Model file for the job. Use its own axes, mm. Coordinates: 2 decimals unless noted, no trailing zeros. Write each loop counter-clockwise with the first axis right and the second up, starting at its lowest first coordinate (ties: lowest second). Pieces come first, ordered by that corner, then holes. Notation, with made-up numbers: M 88.5,33.25 L 133.5,33.25 A24 cw 133.5,65.25 Z; hole C 30.5,26.5 d2. An arc over 180 degrees is marked long. Put each result on its own line as item: value. Start each with the question number.
Q1. Pull direction Z, two halves, no side cores. Call faces 1 (the flat face through (58, 5, 0)), 2 (the cylindrical face through (37.253, -0.902, -0.121)), 3 (the flat face through (-1, 5, 18)): pulls with the +Z half, pulls with the -Z half, needs draft (parallel to the pull), parting line crosses it, or undercut.
Q2. Drop flat-ended pins along their axis: pin 1 (3.5 mm diameter, centred on x = -40, z = 0, fed in from +Y); pin 2 (2 mm diameter, centred on x = 40, y = 6, fed in from -Z). Give the stop position or say it passes through.
Q3. Cut at A-A (z = 0). Write the cut outline in (x, y).
Q4. Cut at C-C (z = -17). Write the cut outline in (x, y), then the cut area to 3 significant figures.
Q5. Drill centre lines: line 1 along X through (y, z) = (-4.75, 0); line 2 along Z through (x, y) = (-40, -2); line 3 along X through (y, z) = (0.5, 2.5). Where is each one in solid material? Low to high.
Q6. Cut at B-B (x = -40). Write the cut outline in (y, z).
Autodesk Inventor part; units mm, degrees
ref_plane "YZ Plane" through (0, 0, 0) normal (1, 0, 0) x (0, 1, 0)
ref_plane "XZ Plane" through (0, 0, 0) normal (0, 1, 0) x (-1, 0, 0)
ref_plane "XY Plane" through (0, 0, 0) normal (0, 0, 1) x (1, 0, 0)
sketch "Sketch1" plane through (0, 0, 0) normal (0, 1, 0) x (-1, 0, 0)
  line L0 (60, 20) -> (-60, 20)
  line L1 (-60, 20) -> (-60, -20)
  line L2 (-60, -20) -> (60, -20)
  line L3 (60, -20) -> (60, 20)
  line L4 (0, 0) -> (-60, 0) construction
  line L5 (0, 0) -> (0, -20) construction
  dimension "d0" = 120
  dimension "d1" = 40
extrude "Extrusion1" add sketch "Sketch1" along normal mid plane 16
sketch "Sketch2" plane through (0, 8, 0) normal (0, 1, 0) x (1, 0, 0)
  line L0 (-60, -20) -> (60, -20)
  line L1 (60, -20) -> (60, 20)
  line L2 (60, 20) -> (-60, 20)
  line L3 (-60, 20) -> (-60, -20)
  circle A0 centre (-40, 0) radius 2.75
  circle A1 centre (40, 0) radius 2.75
  line L4 (-60, 0) -> (60, 0) construction
  line L5 (0, 20) -> (0, -20) construction
  point P0 (0, 0)
  dimension "d5" = 5.5
  dimension "d7" = 40
extrude "Extrusion2" cut sketch "Sketch2" against normal through all contours A0 | A1
chamfer "Chamfer1" distance 5 angle 45 4 edges at (-60, 8, 0) (0, 8, 20) (0, 8, -20) (60, 8, 0)
chamfer "Chamfer2" distance 2 angle 45 2 edges at (-42.75, 8, 0) (37.25, 8, 0)
properties part number "Link" material "MDF Medium Density Fiberboard"
Computed values:
1. face 1: needs draft
1. face 2: undercut
1. face 3: pulls with the +Z half
2. pin 1: through
2. pin 2: z = -18
3. outline: M -60,-8 L -42.75,-8 L -42.75,6 L -44.75,8 L -55,8 L -60,3 Z; M -37.25,-8 L 37.25,-8 L 37.25,6 L 35.25,8 L -35.25,8 L -37.25,6 Z; M 42.75,-8 L 60,-8 L 60,3 L 55,8 L 44.75,8 L 42.75,6 Z
4. outline: M -60,-8 L 60,-8 L 60,3 L 57,6 L -57,6 L -60,3 Z
4. area: 1,670 mm2
5. line 1: -60 to -42.75, -37.25 to 37.25, 42.75 to 60
5. line 2: -20 to -2.75, 2.75 to 20
5. line 3: -60 to -41.15, -38.85 to 38.85, 41.15 to 60
6. outline: M -8,-20 L 3,-20 L 8,-15 L 8,-4.75 L 6,-2.75 L -8,-2.75 Z; M -8,2.75 L 6,2.75 L 8,4.75 L 8,15 L 3,20 L -8,20 Z
